from build123d import *

# Parameters (mm, degrees)
EXTRUDE_2_DEPTH     = 0.5
SKETCH_6_R          = 0.5
CUT_EXTRUDE_1_DEPTH = 8.917160087
EXTRUDE_3_DEPTH     = 1
EXTRUDE_4_DEPTH     = 1
EXTRUDE_5_DEPTH     = 0.4
EXTRUDE_6_DEPTH     = 7.1
SKETCH_11_W         = 4.5
SKETCH_11_H         = 6
CUT_EXTRUDE_2_DEPTH = 0.3
SKETCH_13_W         = 4.5
SKETCH_13_H         = 6
CUT_EXTRUDE_3_DEPTH = 0.3
CUT_EXTRUDE_4_DEPTH = 13.769942202
FILLET_2_R          = 0.5


with BuildPart() as part:
    # 草图5 → 凸台-拉伸2 (new body)
    with BuildSketch(Plane.XY):
        with BuildLine():
            Line((-5.742331288, 1.5), (6.257668712, 1.5))
            ThreePointArc((6.257668712, 1.5), (7.757668712, 0), (6.257668712, -1.5))
            Line((6.257668712, -1.5), (-5.742331288, -1.5))
            ThreePointArc((-5.742331288, -1.5), (-7.242331288, 0), (-5.742331288, 1.5))
        make_face()
    extrude(amount=EXTRUDE_2_DEPTH)

    # 草图6 → 切除-拉伸1 (cut, through all)
    with BuildSketch(Plane(origin=(0, 0, 0), x_dir=(-1, 0, 0), z_dir=(0, 0, -1))):
        with Locations((-6.26778509, 0)):
            Circle(SKETCH_6_R)
    extrude(amount=-CUT_EXTRUDE_1_DEPTH, mode=Mode.SUBTRACT)

    # 草图7 → 凸台-拉伸3 (add)
    with BuildSketch(Plane.XY.offset(0.5)):
        with BuildLine():
            Line((3.97045961, -0.65), (-4.02954039, -0.65))
            ThreePointArc((-4.02954039, -0.65), (-4.67954039, 0), (-4.02954039, 0.65))
            Line((-4.02954039, 0.65), (3.97045961, 0.65))
            ThreePointArc((3.97045961, 0.65), (4.62045961, 0), (3.97045961, -0.65))
        make_face()
    extrude(amount=EXTRUDE_3_DEPTH)

    # 草图8 → 凸台-拉伸4 (add)
    with BuildSketch(Plane.XY.offset(1.5)):
        with BuildLine():
            Line((3, -0.4), (-3, -0.4))
            ThreePointArc((-3, -0.4), (-3.4, 0), (-3, 0.4))
            Line((-3, 0.4), (3, 0.4))
            ThreePointArc((3, 0.4), (3.4, 0), (3, -0.4))
        make_face()
    extrude(amount=EXTRUDE_4_DEPTH)

    # 草图9 → 凸台-拉伸5 (add)
    with BuildSketch(Plane.XY.offset(2.5)):
        with BuildLine():
            Line((-4.050467807, 0.65), (3.949532193, 0.65))
            ThreePointArc((3.949532193, 0.65), (4.599532193, 0), (3.949532193, -0.65))
            Line((3.949532193, -0.65), (-4.050467807, -0.65))
            ThreePointArc((-4.050467807, -0.65), (-4.700467807, 0), (-4.050467807, 0.65))
        make_face()
    extrude(amount=EXTRUDE_5_DEPTH)

    # 草图10 → 凸台-拉伸6 (add)
    with BuildSketch(Plane.XY.offset(2.9)):
        with BuildLine():
            Line((-3, 0.5), (3, 0.5))
            ThreePointArc((3, 0.5), (3.5, 0), (3, -0.5))
            Line((3, -0.5), (-3, -0.5))
            ThreePointArc((-3, -0.5), (-3.5, 0), (-3, 0.5))
        make_face()
    extrude(amount=EXTRUDE_6_DEPTH)

    # 草图11 → 切除-拉伸2 (cut)
    with BuildSketch(Plane(origin=(0, -0.5, 0), x_dir=(-1, 0, 0), z_dir=(0, -1, 0))):
        with Locations((0, -6.5)):
            Rectangle(SKETCH_11_W, SKETCH_11_H)
    extrude(amount=-CUT_EXTRUDE_2_DEPTH, mode=Mode.SUBTRACT)

    # 草图13 → 切除-拉伸3 (cut)
    with BuildSketch(Plane(origin=(0, 0.5, 0), x_dir=(1, 0, 0), z_dir=(0, 1, 0))):
        with Locations((0, -6.5)):
            Rectangle(SKETCH_13_W, SKETCH_13_H)
    extrude(amount=-CUT_EXTRUDE_3_DEPTH, mode=Mode.SUBTRACT)

    # 草图14 → 切除-拉伸4 (cut, through all)
    with BuildSketch(Plane(origin=(0, 0.2, 0), x_dir=(1, 0, 0), z_dir=(0, 1, 0))):
        with BuildLine():
            Line((1.297759643, -5), (-1.297759643, -5))
            ThreePointArc((-1.297759643, -5), (-1.797759643, -4.5), (-1.297759643, -4))
            Line((-1.297759643, -4), (1.297759643, -4))
            ThreePointArc((1.297759643, -4), (1.797759643, -4.5), (1.297759643, -5))
        make_face()
        with BuildLine():
            Line((1.297759643, -8.5), (-1.297759643, -8.5))
            ThreePointArc((-1.297759643, -8.5), (-1.797759643, -8), (-1.297759643, -7.5))
            Line((-1.297759643, -7.5), (1.297759643, -7.5))
            ThreePointArc((1.297759643, -7.5), (1.797759643, -8), (1.297759643, -8.5))
        make_face()
    extrude(amount=-CUT_EXTRUDE_4_DEPTH, mode=Mode.SUBTRACT)

    # 圆角2
    fillet_2_edges = [part.edges().sort_by_distance(p)[0] for p in [
        (-7.242331288, 0, 0),
        (0.257668712, 1.5, 0),
        (7.757668712, 0, 0),
        (0.257668712, -1.5, 0),
    ]]
    fillet(fillet_2_edges, radius=FILLET_2_R - 0.0001)  # a hair under: the kernel refuses the full size


solid = part.part
Design review of the part built by this model. Coordinates are the model's own, in mm. A direction names the side the tool comes from. Coordinates: 2 decimals unless noted, no trailing zeros. Loops run counter-clockwise (first coordinate to the right, second up) from the corner with the lowest first, then second, coordinate; pieces in that order, holes last. Notation, with made-up numbers: M 71.25,47 L 116.25,47 A31 ccw 116.25,77 Z; hole C 11.5,62.5 d10. An arc over 180 degrees is marked long. Answer as CSV lines item,"result".
Item 1: The part is to be moulded in two halves that separate along X. For faces 1 (the face through (-4.68, -0.01, 0.99)), 2 (the face through (0, 0, 10)), 3 (the face through (4.62, 0.01, 0.99)), 4 (the face through (6.767, 0.022, 0.246)), say which applies: pulls with the +X half, pulls with the -X half, needs draft (parallel to the pull), parting line crosses it, or undercut.
Answer list:
face 1,"pulls with the -X half"
face 2,"needs draft"
face 3,"pulls with the +X half"
face 4,"undercut"
Item 2: For P1, Ø2, axis at x = -0.5, z = 5, coming from the -Y side; P2, Ø3, axis at x = -5.5, z = 3, coming from the +Y side; P3, Ø6, axis at x = -0.5, z = 4, coming from the -Y side, all flat-tipped, find the tip position at first contact; note any pin that passes through.
Answer list:
P1,"y = -0.2"
P2,"y = 0.65"
P3,"y = -0.65"
Item 3: Machinability: for faces 5 (the face through (0, -0.65, 1)), 6 (the face through (2.6, 0.5, 6.4)), 7 (the face through (0, -0.2, 6)), which of the approach directions +Z, -Z, +X, -X, +Y, -Y give a long, thin tool a straight path to every point of the face, cutting with its end or side? Answer none if there is none.
Answer list:
face 5,"+Z, +X, -X, -Y"
face 6,"+Z, +X, -X, +Y"
face 7,"-Y"
Item 4: Add section B-B on z = 8. State the section outline as (x, y) points, plus the area to 3 significant figures.
Answer list:
outline,"M -3,-0.5 L -2.25,-0.5 L -2.25,-0.2 L -1.8,-0.2 L -1.8,0.2 L -2.25,0.2 L -2.25,0.5 L -3,0.5 A0.5 ccw Z; M 1.8,-0.2 L 2.25,-0.2 L 2.25,-0.5 L 3,-0.5 A0.5 ccw 3,0.5 L 2.25,0.5 L 2.25,0.2 L 1.8,0.2 Z"
area,"2.65 mm²"
Item 5: For probe 1 along Z at (x, y) = (3.5, 0.55); probe 2 along Y at (x, z) = (1.5, 6.75); probe 3 along Z at (x, y) = (-4, 0.75), list the stretches that pass through material, from the lowest coordinate up.
Answer list:
probe 1,"0 to 1.5, 2.5 to 2.9"
probe 2,"-0.2 to 0.2"
probe 3,"0 to 0.5"
Item 6: Add section A-A on y = 0. Count the separate pieces of the cut face and the enclosed holes in it, plus the area to 3 significant figures.
Answer list:
separate pieces,"2"
enclosed holes,"2"
area,"69.7 mm²"
